```python
from build123d import *

# Parameters (mm, degrees)
SKETCH_1_R          = 1.5
SKETCH_1_R_2        = 4
SKETCH_1_R_3        = 1.7
EXTRUDE_1_DEPTH     = 2
SKETCH_2_R          = 1.65
CUT_EXTRUDE_1_DEPTH = 102.407591669


with BuildPart() as part:
    # Эскиз1 → Бобышка-Вытянуть1 (new body)
    with BuildSketch(Plane(origin=(0, 0, 0), x_dir=(1, 0, 0), z_dir=(0, 1, 0))):
        with BuildLine():
            Line((53.10140272, -1.919174262), (23.610564566, 64.870923375))
            add(Edge.make_bspline(
                [(23.610564566, 64.870923375), (17.392407438, 79.302147967), (7, 83.580680649)],
                knots=[2.190316087, 2.190316087, 2.190316087, 2.897805715, 2.897805715, 2.897805715], degree=2, weights=[1, 0.938082041, 1]))
            Line((7, 83.580680649), (7, 75.655170705))
            add(Edge.make_bspline(
                [(11.648024248, 2.885053055), (46.572977066, 48.339095994), (7, 75.655170705)],
                knots=[3.729556348, 3.729556348, 3.729556348, 5.943348398, 5.943348398, 5.943348398], degree=2, weights=[1, 0.447439597, 1]))
            ThreePointArc((11.648024248, 2.885053055), (-2.842752582, 11.658420037), (-11.66866221, -2.800414652))
            Line((-11.66866221, -2.800414652), (-34.753025964, -12.641731973))
            ThreePointArc((-34.753025964, -12.641731973), (-30.555954815, -49.745776402), (3.465216083, -65.136859857))
            ThreePointArc((3.465216083, -65.136859857), (29.374152775, -58.240684948), (50.320473487, -41.505038039))
            ThreePointArc((50.320473487, -41.505038039), (57.298081669, -22.104606133), (53.10140272, -1.919174262))
        make_face()
        with Locations(Location((9.550649772, -54.164426416, 0), (0, 0, 270))):
            Circle(SKETCH_1_R, mode=Mode.SUBTRACT)
        with Locations(Location((31.546703999, -45.053362436, 0), (0, 0, 90))):
            Circle(SKETCH_1_R, mode=Mode.SUBTRACT)
        with Locations(Location((0, 0, 0), (0, 0, 270))):
            Circle(SKETCH_1_R_2, mode=Mode.SUBTRACT)
        with Locations(Location((0, -9, 0), (0, 0, 270))):
            Circle(SKETCH_1_R_3, mode=Mode.SUBTRACT)
        with Locations(Location((-7.794228634, 4.5, 0), (0, 0, 270))):
            Circle(SKETCH_1_R_3, mode=Mode.SUBTRACT)
        with Locations(Location((7.794228634, 4.5, 0), (0, 0, 270))):
            Circle(SKETCH_1_R_3, mode=Mode.SUBTRACT)
        with BuildLine():
            Line((5.20136166, -10.814149845), (31.546703999, 1.857364378))
            ThreePointArc((31.546703999, 1.857364378), (43.724501128, -16.162599301), (36.769552622, -36.769552622))
            ThreePointArc((36.769552622, -36.769552622), (19.899538483, -48.041735691), (0, -52))
            ThreePointArc((0, -52), (-18.737913487, -43.284188232), (-24.14389825, -23.338008012))
            Line((-24.14389825, -23.338008012), (4.70602312, -11.038720324))
            ThreePointArc((4.70602312, -11.038720324), (4.95496481, -10.929241681), (5.20136166, -10.814149845))
        make_face(mode=Mode.SUBTRACT)
    extrude(amount=EXTRUDE_1_DEPTH)

    # Эскиз2 → Вырез-Вытянуть1 (cut, through all)
    with BuildSketch(Plane.XZ):
        with Locations(Location((22.937226804, -23.75718593, 0), (0, 0, 270))):
            Circle(SKETCH_2_R)
        with Locations(Location((15.797221102, -70.877249978, 0), (0, 0, 270))):
            Circle(SKETCH_2_R)
        with Locations(Location((22.937226804, -50.24281407, 0), (0, 0, 270))):
            Circle(SKETCH_2_R)
    extrude(amount=-CUT_EXTRUDE_1_DEPTH, mode=Mode.SUBTRACT)


solid = part.part
```
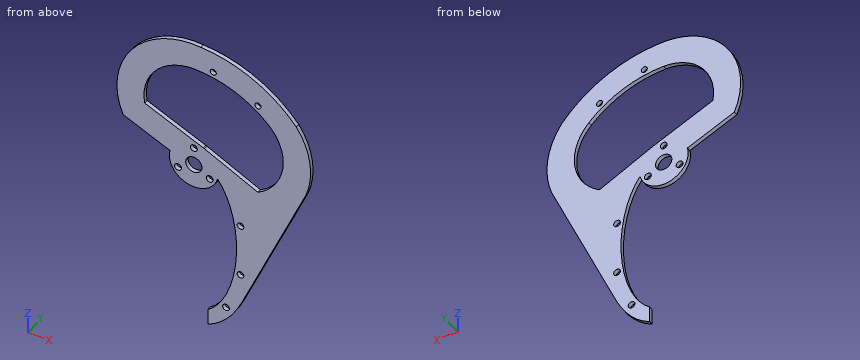
Build history of the part. All positions in model axes, mm. Give positions to 0.01 mm unless a question says otherwise; leave off trailing zeros. Loops run counter-clockwise (first coordinate to the right, second up) from the corner with the lowest first, then second, coordinate; pieces in that order, holes last. Notation, with made-up numbers: (64, 69) -> (108, 69) arc R20 cw to (108, 91) -> close; hole circle Ø5 at (28, 29). An arc over 180 degrees is marked (long way). One line per question, with ' | ' between items.
Q1. Drop a flat-ended pin along its axis: pin 1 (2 mm diameter, centred on x = 22.94, z = -23.76, fed in from -Y). Give the stop position or say it passes through.
Filled sheet:
pin 1: passes through
Q2. Cut at C-C, the plane y = 0.9. Count the separate pieces of the cut face and the enclosed holes in it, plus the area to 3 significant figures.
Filled sheet:
separate pieces: 1 | enclosed holes: 10 | area: 4,150 mm²
Q3. Cut at A-A, the plane z = 0. Write the cut outline in (x, y), plus the area to 3 significant figures.
Filled sheet:
outline: (-12, 0) -> (-4, 0) -> (-4, 2) -> (-12, 2) -> close; (4, 0) -> (27.69, 0) -> (27.69, 2) -> (4, 2) -> close; (34.35, 0) -> (52.25, 0) -> (52.25, 2) -> (34.35, 2) -> close | area: 99.2 mm²
Q4. Drill centre lines: line 1 along Z through (x, y) = (12.5, 1.35); line 2 along X through (y, z) = (1.25, -1); line 3 along Z through (x, y) = (24, 0.2). Where is each one in solid material? Low to high. Write a range as [from, to].
Filled sheet:
line 1: z = [-80.31, -69.95], [-4.05, 7.3], [50.48, 64.02] | line 2: x = [-11.96, -3.87], [3.87, 29.76], [32.94, 51.81] | line 3: z = [-63.99, -51.5], [-48.98, -25.02], [-22.5, 1.77], [46.13, 60.65]
Q5. Cut at B-B, the plane x = -17. Write the cut outline in (y, z), plus the area to 3 significant figures.
Filled sheet:
outline: (0, 5.07) -> (2, 5.07) -> (2, 20.29) -> (0, 20.29) -> close; (0, 45.14) -> (2, 45.14) -> (2, 61.26) -> (0, 61.26) -> close | area: 62.7 mm²
